Work out the finished part from the listing and answer in its coordinate system (mm). Coordinates: 2 decimals unless noted, no trailing zeros. Write each loop counter-clockwise with the first axis right and the second up, starting at its lowest first coordinate (ties: lowest second). Pieces come first, ordered by that corner, then holes. Notation, with made-up numbers: M 10.25,13 L 45.25,13 A6 cw 45.25,24 Z; hole C 75.5,21 d11. An arc over 180 degrees is marked long. Answer as CSV lines item,"result". Start each with the question number.
(1) Flat-ended cylindrical pins translate along their axes: P1, Ø12, axis at x = 426, y = -31, coming from the +Z side; P2, Ø2, axis at x = 293, y = -2.5, coming from the +Z side; P3, Ø4, axis at y = -13, z = 96, coming from the -X side. Find the tip coordinate at first contact, or state that the pin passes through.
(2) A cutting plane is placed at C-C on z = 99. Count the separate pieces of the cut face and the enclosed holes in it, then the cut area to 3 significant figures.
(3) A cutting plane is placed at B-B on x = 404.5. Give the vertices of the cut face in (y, z).
(4) Find the intervals of material crossed by L1, parallel to Y at x = 284, z = 95.75; L2, parallel to X at y = 0, z = 98.75; L3, parallel to Z at x = 260.5, y = -11, in increasing order. Write a range as [from, to].
(5) A cutting plane is placed at A-A on x = 369. Give the vertices of the cut face in (y, z), then the cut area to 3 significant figures.
from build123d import *

# Parameters (mm, degrees)
SKETCH1_W           = 6.35
SKETCH1_H           = 19.05
BOSS_EXTRUDE1_DEPTH = 6.35
CUT_EXTRUDE1_DEPTH  = 6.35
EXTRUDE_THIN3_START = -6.35
EXTRUDE_THIN3_DEPTH = 6.35
FILLET2_R           = 2.54


with BuildPart() as part:
    # Sketch1 → Boss-Extrude1 (new body)
    with BuildSketch(Plane(origin=(-0.338050957, -2.166981544, 94.101832391), x_dir=(0.999993551, -8.2681e-05, 0.003590468), z_dir=(-0.00359142, -0.023021797, 0.999728512))):
        with BuildLine():
            Line((243.227078617, -9.06878027), (243.227078617, -28.11878027))
            Line((243.227078617, -28.11878027), (243.227078617, -33.122710711))
            Line((243.227078617, -33.122710711), (455.95107602, -33.122710711))
            Line((455.95107602, -33.122710711), (455.95107602, -28.298303458))
            Line((455.95107602, -28.298303458), (455.951838068, -9.248303458))
            Line((455.951838068, -9.248303458), (455.952670896, 11.571066175))
            Line((455.952670896, 11.571066175), (455.928271144, 11.571065016))
            Line((455.928271144, 11.571065016), (356.413957438, 11.566336687))
            add(Edge.make_bspline(
                [(356.413957438, 11.566336687), (356.413154179, 10.230187882), (356.307050724, 8.928363908), (356.110746239, 7.669666942)],
                knots=[0.928343353, 0.928343353, 0.928343353, 0.928343353, 1, 1, 1, 1], degree=3, weights=[0.866956056, 0.907880921, 0.952228902, 1]))
            Line((356.110746239, 7.669666942), (356.069707191, 7.406526111))
            add(Edge.make_bspline(
                [(356.069707191, 7.406526111), (349.645197224, -33.787190013), (305.128556412, -35.346859606), (305.574396885, 11.563921094)],
                knots=[0, 0, 0, 0, 0.932216201, 0.932216201, 0.932216201, 0.932216201], degree=3, weights=[1, 0.378522533, 0.336396429, 0.873621689]))
            Line((305.574396885, 11.563921094), (243.227078617, 11.56095872))
            Line((243.227078617, 11.56095872), (243.227078617, -9.06878027))
        make_face()
        with Locations((240.052078617, -18.59378027)):
            Rectangle(SKETCH1_W, SKETCH1_H)
        Polygon((455.951838068, -9.248303458), (455.95107602, -28.298303458), (462.301838068, -28.298303458), (462.301838068, -9.248303458), align=None)
    extrude(amount=BOSS_EXTRUDE1_DEPTH)

    # Sketch4 → Cut-Extrude1 (cut)
    with BuildSketch(Plane(origin=(-0.360856472, -2.313169952, 100.450108445), x_dir=(0.999993551, -8.2681e-05, 0.003590468), z_dir=(-0.00359142, -0.023021797, 0.999728512))):
        with BuildLine():
            Line((447.06107602, -24.232710711), (447.061359456, -21.212677023))
            Line((447.061359456, -21.212677023), (447.062315249, 2.680643748))
            Line((447.062315249, 2.680643748), (364.155660196, 2.676704517))
            add(Edge.make_bspline(
                [(364.155660196, 2.676704517), (363.682655748, 0.861202633), (363.064243452, -0.90556276), (361.917066697, -3.482121278), (361.496667699, -4.330871885), (360.585218077, -5.993055638), (360.098114328, -6.79975573), (358.545391798, -9.148799286), (357.388958371, -10.620549815), (355.471920122, -12.686399888), (354.802074961, -13.351532301), (353.400459371, -14.63170826), (352.678029759, -15.238263747), (350.447885909, -16.96045064), (348.877725006, -17.979235773), (347.099980812, -18.935765266), (346.975195928, -19.001918677), (346.849935868, -19.067335155)],
                knots=[0, 0, 0, 0, 0.0625, 0.0625, 0.09375, 0.09375, 0.125, 0.125, 0.1875, 0.1875, 0.21875, 0.21875, 0.25, 0.25, 0.3125, 0.3125, 0.317199008, 0.317199008, 0.317199008, 0.317199008], degree=3))
            Line((346.849935868, -19.067335155), (346.849935868, -24.232710711))
            Line((346.849935868, -24.232710711), (447.06107602, -24.232710711))
        make_face()
        with BuildLine():
            Line((252.117078617, -24.232710711), (315.099935868, -24.232710711))
            Line((315.099935868, -24.232710711), (315.099935868, -19.067335155))
            add(Edge.make_bspline(
                [(315.099935868, -19.067335155), (314.975929033, -19.002569071), (314.852285143, -18.937030581), (313.903603629, -18.426757245), (313.094537504, -17.948032357), (311.509855263, -16.919395321), (310.733380771, -16.36830218), (308.497317264, -14.638176011), (307.115550753, -13.373897611), (305.203441753, -11.314112149), (304.592963657, -10.600151869), (303.426963523, -9.116307482), (302.869814737, -8.343419981), (301.312262481, -5.982806196), (300.415072454, -4.342556455), (298.894695177, -0.932977765), (298.271468298, 0.836332514), (297.792394207, 2.673551329)],
                knots=[0.682832517, 0.682832517, 0.682832517, 0.682832517, 0.6875, 0.6875, 0.71875, 0.71875, 0.75, 0.75, 0.8125, 0.8125, 0.84375, 0.84375, 0.875, 0.875, 0.9375, 0.9375, 1, 1, 1, 1], degree=3))
            Line((297.792394207, 2.673551329), (252.117078617, 2.67138111))
            Line((252.117078617, 2.67138111), (252.117078617, -24.232710711))
        make_face()
    extrude(amount=-CUT_EXTRUDE1_DEPTH, mode=Mode.SUBTRACT)

    # Sketch5 → Extrude-Thin3 (add)
    with BuildSketch(Plane(origin=(-0.360856472, -2.313169952, 100.450108445), x_dir=(0.999993551, -8.2681e-05, 0.003590468), z_dir=(-0.00359142, -0.023021797, 0.999728512)).offset(EXTRUDE_THIN3_START)):
        Polygon((250.180703918, 1.027588841), (274.956201281, -28.157757229), (299.728925104, 1.029943078), (295.85586331, 4.317159581), (274.955828291, -20.307664192), (254.053453316, 4.31517338), align=None)
        Polygon((362.38371865, 0.856862997), (391.792672106, -27.778018594), (419.426789837, -0.86614126), (445.288961546, -26.052383839), (448.833190494, -22.413037583), (419.426789837, 6.224802604), (391.792335202, -20.687402828), (365.927601742, 4.496546037), align=None)
    extrude(amount=EXTRUDE_THIN3_DEPTH)

    # Fillet2
    fillet2_edges = [part.edges().sort_by_distance(p)[0] for p in [
        (298.32854124, -2.470729974, 98.343628252),
        (255.097636261, 0.409634721, 98.254654941),
        (294.109382675, 0.408262278, 98.394768941),
        (251.765998957, -3.514034664, 98.152331935),
        (271.273016149, -26.488822109, 97.693344331),
        (274.60460134, -22.565091347, 97.795668563),
        (277.936290782, -26.489373041, 97.717268759),
        (362.969132405, -2.325780207, 98.579180702),
        (443.068140014, -26.503026473, 98.310173185),
        (395.081122323, -26.49905881, 98.137876228),
        (446.709043574, -22.959091678, 98.404862651),
        (367.44463473, 0.405682327, 98.658158726),
        (415.433854418, 0.403994055, 98.830516083),
        (391.440354753, -22.95438955, 98.206423967),
        (422.715052674, 0.4037379, 98.856667125),
        (419.074631168, -3.140666269, 98.761968583),
        (387.79956879, -26.498456757, 98.111731875),
        (314.748450021, -21.32841022, 97.968359479),
        (314.748450021, -26.492416744, 97.849442487),
        (251.765998957, -26.487209229, 97.623304561),
        (446.709978354, 0.402893753, 98.942846938),
        (346.49824526, -26.495041881, 97.963439843),
        (346.49824526, -21.331035356, 98.082356835),
    ]]
    fillet(fillet2_edges, radius=FILLET2_R)


solid = part.part
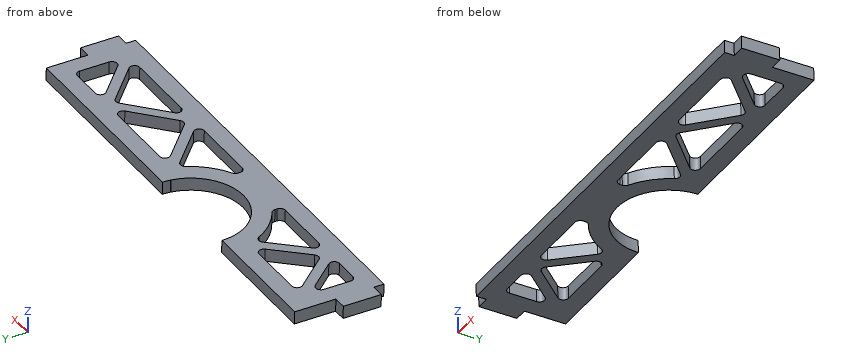
Here are the results:
1,P1,"stops at z = 101.44"
1,P2,"stops at z = 101.52"
1,P3,"stops at x = 236.53"
2,separate pieces,"1"
2,enclosed holes,"7"
2,area,"5,810 mm^2"
3,outline,"M -35.46,101.14 L -35.31,94.79 L -26.43,95 L -26.57,101.35 Z; M -17.39,101.56 L -17.27,95.21 L -10.18,95.37 L -10.3,101.72 Z; M 0.33,101.97 L 0.48,95.62 L 9.37,95.82 L 9.22,102.17 Z"
4,L1,"y = [-35.34, -26.44], [-19.31, -11.46], [0.47, 9.36]"
4,L2,"x = [242.87, 259.22], [289.99, 306.89], [354.35, 372.32], [410.56, 427.59], [445.55, 455.6]"
4,L3,"z = [94.84, 101.19]"
5,outline,"M -35.46,101.01 L -35.31,94.67 L -26.42,94.87 L -26.57,101.22 Z; M -8.28,101.64 L -8.11,95.29 L 9.37,95.69 L 9.22,102.04 Z"
5,area,"168 mm^2"
